Autodesk Inventor part; units mm, degrees
ref_plane "YZ Plane" through (0, 0, 0) normal (1, 0, 0) x (0, 1, 0)
ref_plane "XZ Plane" through (0, 0, 0) normal (0, 1, 0) x (-1, 0, 0)
ref_plane "XY Plane" through (0, 0, 0) normal (0, 0, 1) x (1, 0, 0)
sketch "Sketch1" plane through (0, 0, 0) normal (0, 1, 0) x (-1, 0, 0)
  line L0 (0, 0) -> (-30, 0)
  line L1 (-30, 0) -> (-30, 30)
  line L2 (-30, 30) -> (-115, 30)
  line L3 (-115, 30) -> (-115, 0)
  line L4 (-115, 0) -> (-145, 0)
  line L5 (0, 3) -> (-27, 3)
  line L6 (-27, 3) -> (-27, 33)
  line L7 (-27, 33) -> (-118, 33)
  line L8 (-118, 33) -> (-118, 3)
  line L9 (-118, 3) -> (-145, 3)
  line L10 (0, 0) -> (0, 3)
  line L11 (-145, 0) -> (-145, 3)
  dimension "d0" = 30
  dimension "d1" = 30
  dimension "d2" = 3
  dimension "d28" = 85
extrude "Extrusion1" add sketch "Sketch1" along normal blind 82
sketch "Sketch2" plane through (27, 0, 33) normal (0, 0, 1) x (1, 0, 0)
  line L0 (0, 82) -> (91, 82)
  line L1 (45.5, 82) -> (45.5, 0) construction
  line L2 (0, 0) -> (91, 0)
  circle A0 centre (45.5, 41) radius 32.5 construction
  line L3 (45.5, 41) -> (68.481, 63.981) construction
  circle A1 centre (68.481, 63.981) radius 3.05
  circle A2 centre (22.519, 63.981) radius 3.05
  circle A3 centre (22.519, 18.019) radius 3.05
  circle A4 centre (68.481, 18.019) radius 3.05
  circle A5 centre (45.5, 41) radius 25.0125
  point P0 (-27, 0)
  dimension "d6" = 65
  dimension "d7" = 6.1
  dimension "d8" = 45
  dimension "d11" = 360
  dimension "d15" = 50.025
extrude "Extrusion2" cut sketch "Sketch2" against normal blind 82
sketch "Sketch3" plane through (0, 0, 3) normal (0, 0, 1) x (1, 0, 0)
  circle A0 centre (72.5, 41) radius 25.0125 construction
  line L0 (12.5, 66) -> (132.5, 66) construction
  line L1 (132.5, 66) -> (132.5, 16) construction
  line L2 (132.5, 16) -> (12.5, 16) construction
  line L3 (12.5, 16) -> (12.5, 66) construction
  line L4 (12.5, 66) -> (132.5, 16) construction
  line L5 (132.5, 66) -> (12.5, 16) construction
  circle A1 centre (12.5, 66) radius 3.05
  circle A2 centre (12.5, 16) radius 3.05
  circle A3 centre (132.5, 66) radius 3.05
  circle A4 centre (132.5, 16) radius 3.05
  dimension "d29" = 6.1
  dimension "d30" = 120
  dimension "d31" = 50
extrude "Extrusion3" cut sketch "Sketch3" against normal blind 10
properties part number "TopMotorBracket"
For this review, take the finished solid that the model builds, in its own axes (mm). A direction names the side the tool comes from. Round coordinates to 2 decimals unless told otherwise and drop trailing zeros. Order: outer loops, then holes, each group sorted by start corner. A loop starts at its lowest first (then second) coordinate and runs counter-clockwise, first axis right, second up. Notation, with made-up numbers: (-15, 4.25) -> (22, 4.25) arc R20 cw to (22, 41.25) -> close; hole circle Ø9 at (11.25, -32.5). An arc over 180 degrees is marked (long way). Use a Markdown table: item, result.
Item 1: For line 1 along Y through (x, z) = (12.5, 0.95); line 2 along X through (y, z) = (67.5, 7); line 3 along Z through (x, y) = (36, 36), list the stretches that pass through material, from the lowest coordinate up. Write a range as [from, to].
Resolved:
| item | result |
|---|---|
| line 1 | y = [0, 12.95], [19.05, 62.95], [69.05, 82] |
| line 2 | x = [27, 30], [115, 118] |
| line 3 | z = [30, 33] |
Item 2: Draft analysis for pull direction X (two halves, no side actions). For faces 1 (the cylindrical face through (11.839, 63.023, 1.521)), 2 (the cylindrical face through (46.47, 18.15, 31.52)), 3 (the flat face through (73, 0, 31)), 4 (the flat face through (145, 40, 1)), state which applies: +X half, -X half, draft (parallel to the pull), parting line (faces both ways), or undercut.
Resolved:
| item | result |
|---|---|
| face 1 | undercut |
| face 2 | undercut |
| face 3 | draft |
| face 4 | +X half |
Item 3: Take a section at C-C (z = 13.5). State the section outline as (x, y) points, plus the area to 3 significant figures.
Resolved:
| item | result |
|---|---|
| outline | (27, 0) -> (30, 0) -> (30, 82) -> (27, 82) -> close; (115, 0) -> (118, 0) -> (118, 82) -> (115, 82) -> close |
| area | 492 mm² |
Item 4: For pin 1 (1 mm diameter, centred on x = 44.5, y = 12.5, fed in from -Z); pin 2 (3 mm diameter, centred on y = 62, z = 28.5, fed in from -X); pin 3 (9 mm diameter, centred on y = 20.5, z = 13.5, fed in from +X); pin 4 (3.5 mm diameter, centred on x = 12.5, y = 16, fed in from +Z), all flat-tipped, find the tip position at first contact; note any pin that passes through.
Resolved:
| item | result |
|---|---|
| pin 1 | stops at z = 30 |
| pin 2 | stops at x = 27 |
| pin 3 | stops at x = 118 |
| pin 4 | passes through |
Item 5: Take a section at A-A (x = 132.5). State the section outline as (y, z) points.
Resolved:
| item | result |
|---|---|
| outline | (0, 0) -> (12.95, 0) -> (12.95, 3) -> (0, 3) -> close; (19.05, 0) -> (62.95, 0) -> (62.95, 3) -> (19.05, 3) -> close; (69.05, 0) -> (82, 0) -> (82, 3) -> (69.05, 3) -> close |
Item 6: Take a section at B-B (y = 41). State the section outline as (x, z) points, plus the area to 3 significant figures.
Resolved:
| item | result |
|---|---|
| outline | (0, 0) -> (30, 0) -> (30, 30) -> (47.49, 30) -> (47.49, 33) -> (27, 33) -> (27, 3) -> (0, 3) -> close; (97.51, 30) -> (115, 30) -> (115, 0) -> (145, 0) -> (145, 3) -> (118, 3) -> (118, 33) -> (97.51, 33) -> close |
| area | 465 mm² |
Item 7: Take a section at D-D (x = 72.5). State the section outline as (y, z) points, plus the area to 3 significant figures.
Resolved:
| item | result |
|---|---|
| outline | (0, 30) -> (15.99, 30) -> (15.99, 33) -> (0, 33) -> close; (66.01, 30) -> (82, 30) -> (82, 33) -> (66.01, 33) -> close |
| area | 95.9 mm² |
Item 8: Machinability: for faces 5 (the flat face through (0, 40, 1)), 6 (the flat face through (27, 40, 18)), 7 (the flat face through (115, 40, 15)), 8 (the flat face through (131, 40, 3)), which of the approach directions +Z, -Z, +X, -X, +Y, -Y give a long, thin tool a straight path to every point of the face, cutting with its end or side? Answer none if there is none.
Resolved:
| item | result |
|---|---|
| face 5 | +Z, -Z, -X, +Y, -Y |
| face 6 | +Z, -X, +Y, -Y |
| face 7 | -Z, +Y, -Y |
| face 8 | +Z, +X, +Y, -Y |
